from build123d import *

# Parameters (mm, degrees)
SKETCH1_W           = 400
SKETCH1_H           = 435
BOSS_EXTRUDE1_DEPTH = 480
SKETCH4_W           = 350
SKETCH4_H           = 200
CUT_EXTRUDE1_DEPTH  = 300
SHELL1_START        = -180
SHELL1_DEPTH        = 360
SKETCH5_W           = 400
SKETCH5_H           = 435
BOSS_EXTRUDE2_DEPTH = 50
SKETCH3_R           = 160
CUT_EXTRUDE2_DEPTH  = 70
SKETCH6_R           = 42.5
CUT_EXTRUDE3_DEPTH  = 20


# Read off the part's stored shape, not the designer's step: Shell1
with BuildPart() as part:
    # Sketch1 → Boss-Extrude1 (new body)
    with BuildSketch(Plane(origin=(0, 0, 0), x_dir=(1, 0, 0), z_dir=(0, 1, 0))):
        with Locations((0, -93.5)):
            Rectangle(SKETCH1_W, SKETCH1_H)
    extrude(amount=BOSS_EXTRUDE1_DEPTH)

    # Sketch4 → Cut-Extrude1 (cut)
    with BuildSketch(Plane(origin=(0, 0, -124), x_dir=(-1, 0, 0), z_dir=(0, 0, -1))):
        with Locations((0, 125)):
            Rectangle(SKETCH4_W, SKETCH4_H)
    extrude(amount=-CUT_EXTRUDE1_DEPTH, mode=Mode.SUBTRACT)

    # Shell1 outline → Shell1 (cut)
    with BuildSketch(Plane.YZ.offset(SHELL1_START)):
        Polygon((245, -104), (460, -104), (460, 311), (20, 311), (20, 196), (245, 196), align=None)
    extrude(amount=SHELL1_DEPTH, mode=Mode.SUBTRACT)

    # Sketch5 → Boss-Extrude2 (add)
    with BuildSketch(Plane(origin=(0, 480, 0), x_dir=(1, 0, 0), z_dir=(0, 1, 0))):
        with Locations((0, -93.5)):
            Rectangle(SKETCH5_W, SKETCH5_H)
    extrude(amount=BOSS_EXTRUDE2_DEPTH)

    # Sketch3 → Cut-Extrude2 (cut)
    with BuildSketch(Plane(origin=(0, 530, 0), x_dir=(1, 0, 0), z_dir=(0, 1, 0))):
        with Locations(Location((0, -64.5, 0), (0, 0, 270))):
            Circle(SKETCH3_R)
    extrude(amount=-CUT_EXTRUDE2_DEPTH, mode=Mode.SUBTRACT)

    # Sketch6 → Cut-Extrude3 (cut)
    with BuildSketch(Plane(origin=(0, 245, 0), x_dir=(1, 0, 0), z_dir=(0, 1, 0))):
        with Locations(Location((0, 20, 0), (0, 0, 270))):
            Circle(SKETCH6_R)
    extrude(amount=-CUT_EXTRUDE3_DEPTH, mode=Mode.SUBTRACT)


solid = part.part
Design review of the part built by this model. Coordinates are the model's own, in mm. A direction names the side the tool comes from. Give positions to 0.01 mm unless a question says otherwise; leave off trailing zeros. Loops run counter-clockwise (first coordinate to the right, second up) from the corner with the lowest first, then second, coordinate; pieces in that order, holes last. Notation, with made-up numbers: (60.5, 10.25) -> (92.5, 10.25) arc R19 ccw to (92.5, 25.25) -> close; hole circle Ø5 at (-3, -39). An arc over 180 degrees is marked (long way). One line per question, with ' | ' between items. Start each with the question number.
(1) For faces 1 (the face through (200, 261, 97)), 2 (the face through (48.1, 495.5, 217.1)), 3 (the face through (175, 124, 24)), 4 (the face through (180, 286, 153)), list the 3-axis set-ups (+Z, -Z, +X, -X, +Y, -Y) from which the entire face can be reached by the end or side of a thin tool; tool diameter is ignored.
(2) We need section C-C (y = 99). State the section outline as (x, z) points, and give its area (3 significant figures).
(3) We need section B-B (x = 0). State the section outline as (y, z) points.
(4) We need section A-A (z = 265). State the section outline as (x, y) points, and give its area (3 significant figures).
(5) Insertion check: P1, Ø6, axis at x = -24.5, z = 146.5, coming from the +Y side; P2, Ø1.5, axis at x = -124, y = 138.5, coming from the -Z side. Each pin has a flat end and moves straight along its axis. Give the tip position at first contact, or say it passes through.
(6) We need section D-D (x = -75). State the section outline as (y, z) points, and give its area (3 significant figures).
(7) For line 1 (Y direction, x = 135.5, z = 174.5); line 2 (Y direction, x = 169, z = 248.5); line 3 (X direction, y = 486.5, z = 64.5), list the stretches that pass through material, from the lowest coordinate up.
(8) Draft analysis for pull direction Y (two halves, no side actions). For faces 5 (the face through (-3, 245, 48)), 6 (the face through (-175, 124, 24)), 7 (the face through (-200, 261, 97)), 8 (the face through (-3, 0, 90)), state which applies: +Y half, -Y half, draft (parallel to the pull), parting line (faces both ways), or undercut.
The answers:
1) face 1: +Z, -Z, +X, +Y, -Y | face 2: +Y | face 3: -Z | face 4: +Z
2) outline: (-200, -124) -> (-175, -124) -> (-175, 176) -> (175, 176) -> (175, -124) -> (200, -124) -> (200, 311) -> (180, 311) -> (180, 196) -> (-180, 196) -> (-180, 311) -> (-200, 311) -> close | area: 27,600 mm^2
3) outline: (0, -124) -> (25, -124) -> (25, 176) -> (225, 176) -> (225, 22.5) -> (245, 22.5) -> (245, 196) -> (20, 196) -> (20, 311) -> (0, 311) -> close; (225, -124) -> (530, -124) -> (530, -95.5) -> (460, -95.5) -> (460, -104) -> (245, -104) -> (245, -62.5) -> (225, -62.5) -> close; (460, 224.5) -> (530, 224.5) -> (530, 311) -> (460, 311) -> close
4) outline: (-200, 0) -> (200, 0) -> (200, 530) -> (-200, 530) -> close; hole (-180, 20) -> (180, 20) -> (180, 460) -> (-180, 460) -> close | area: 53,600 mm^2
5) P1: stops at y = 245 | P2: stops at z = 176
6) outline: (0, -124) -> (25, -124) -> (25, 176) -> (225, 176) -> (225, -124) -> (530, -124) -> (530, -76.83) -> (460, -76.83) -> (460, -104) -> (245, -104) -> (245, 196) -> (20, 196) -> (20, 311) -> (0, 311) -> close; (460, 205.83) -> (530, 205.83) -> (530, 311) -> (460, 311) -> close | area: 35,700 mm^2
7) line 1: y = 0 to 25, 225 to 245, 460 to 530 | line 2: y = 0 to 20, 460 to 530 | line 3: x = -200 to -160, 160 to 200
8) face 5: undercut | face 6: undercut | face 7: draft | face 8: -Y half
